Here's how the part is built. I have some questions about the finished solid (model axes, mm). A direction names the side the tool comes from. Give positions to 0.01 mm unless a question says otherwise; leave off trailing zeros. Loops run counter-clockwise (first coordinate to the right, second up) from the corner with the lowest first, then second, coordinate; pieces in that order, holes last. Notation, with made-up numbers: (29.25, 79.25) - (35.25, 79.25) arc R10 cw to (35.25, 97.25) - close; hole circle Ø5 at (42.5, 19.25). An arc over 180 degrees is marked (long way). Use one line per item in the form item = value.
from build123d import *


with BuildPart() as part:
    # Sketch1 → Pasador_codo (revolve)
    with BuildSketch(Plane.XY, mode=Mode.PRIVATE) as pasador_codo_sk:
        Polygon((-14, 0), (-14, 4.5), (-12.5, 4.5), (-12.5, 3), (34, 3), (34, 4.5), (35.5, 4.5), (35.5, 0), align=None)
    revolve(pasador_codo_sk.sketch.rotate(Axis((-18, 0, 0), (1, 0, 0)), 90), axis=Axis((-18, 0, 0), (1, 0, 0)))


solid = part.part
(1) For P1, Ø5, axis at x = -5, z = 3.5, coming from the -Y side; P2, Ø1, axis at x = 9, y = -1, coming from the +Z side; P3, Ø4, axis at x = 22, z = -1, coming from the +Y side, each with a flat end and sliding along its axis, tell me the tip position at first contact or that it passes through.
Geometry says:
P1 = -2.83
P2 = 2.96
P3 = 3
(2) If we section it at A-A (z = 3.75): List the corners of the cut face in (x, y) for me.
Geometry says:
outline = (-14, -2.49) - (-12.5, -2.49) - (-12.5, 2.49) - (-14, 2.49) - close; (34, -2.49) - (35.5, -2.49) - (35.5, 2.49) - (34, 2.49) - close
(3) If we section it at B-B (y = 3.5): List the corners of the cut face in (x, z) for me.
Geometry says:
outline = (-14, -2.83) - (-12.5, -2.83) - (-12.5, 2.83) - (-14, 2.83) - close; (34, -2.83) - (35.5, -2.83) - (35.5, 2.83) - (34, 2.83) - close
(4) If we section it at D-D (y = 0): List the corners of the cut face in (x, z) for me, plus the area to 3 significant figures.
Geometry says:
outline = (-14, -4.5) - (-12.5, -4.5) - (-12.5, -3) - (34, -3) - (34, -4.5) - (35.5, -4.5) - (35.5, 4.5) - (34, 4.5) - (34, 3) - (-12.5, 3) - (-12.5, 4.5) - (-14, 4.5) - close
area = 306 mm²
(5) For faces 1 (the flat face through (-14, 0, 0)), 2 (the cylindrical face through (11.08, -0.9, 2.86)), which set-ups out of +Z, -Z, +X, -X, +Y, -Y let a thin tool reach every point of the face, with its end or its side?
Geometry says:
face_1 = +Z, -Z, -X, +Y, -Y
face_2 = none
(6) If we section it at C-C (z = 1): List the corners of the cut face in (x, y) for me.
Geometry says:
outline = (-14, -4.39) - (-12.5, -4.39) - (-12.5, -2.83) - (34, -2.83) - (34, -4.39) - (35.5, -4.39) - (35.5, 4.39) - (34, 4.39) - (34, 2.83) - (-12.5, 2.83) - (-12.5, 4.39) - (-14, 4.39) - close
(7) If I drill on probe 1 along X at (y, z) = (-0.25, -4); probe 2 along Z at (x, y) = (-7.5, -1.25); probe 3 along Z at (x, y) = (7.5, 2.25), over which ranges is the centre line in solid material (lowest first)?
Geometry says:
probe_1 = -14 to -12.5, 34 to 35.5
probe_2 = -2.73 to 2.73
probe_3 = -1.98 to 1.98
